```python
from build123d import *

# Parameters (mm, degrees)
SKETCH1_R           = 46.609
BOSS_EXTRUDE1_DEPTH = 38.1
SKETCH2_R           = 1.27
CUT_EXTRUDE1_DEPTH  = 38.1
SKETCH3_R           = 8.89
CUT_EXTRUDE2_DEPTH  = 38.1
SKETCH4_W           = 33.02
SKETCH4_H           = 33.02
CUT_EXTRUDE3_DEPTH  = 19.05
FILLET1_R           = 5.08


with BuildPart() as part:
    # Sketch1 → Boss-Extrude1 (new body)
    with BuildSketch(Plane(origin=(0, 0, 0), x_dir=(1, 0, 0), z_dir=(0, 1, 0))):
        Circle(SKETCH1_R)
    extrude(amount=BOSS_EXTRUDE1_DEPTH)

    # Sketch2 → Cut-Extrude1 (cut)
    with BuildSketch(Plane(origin=(0, 38.1, 0), x_dir=(1, 0, 0), z_dir=(0, 1, 0))):
        with Locations((12.7, 32.512)):
            Circle(SKETCH2_R)
        with Locations((-12.7, 32.512)):
            Circle(SKETCH2_R)
    extrude(amount=-CUT_EXTRUDE1_DEPTH, mode=Mode.SUBTRACT)

    # Sketch3 → Cut-Extrude2 (cut)
    with BuildSketch(Plane(origin=(0, 38.1, 0), x_dir=(1, 0, 0), z_dir=(0, 1, 0))):
        with Locations((-26.409958794, 0)):
            Circle(SKETCH3_R)
    extrude(amount=-CUT_EXTRUDE2_DEPTH, mode=Mode.SUBTRACT)

    # Sketch4 → Cut-Extrude3 (cut)
    with BuildSketch(Plane(origin=(0, 38.1, 0), x_dir=(1, 0, 0), z_dir=(0, 1, 0))):
        with Locations((16.51, 0)):
            Rectangle(SKETCH4_W, SKETCH4_H)
    extrude(amount=-CUT_EXTRUDE3_DEPTH, mode=Mode.SUBTRACT)

    # Fillet1
    fillet1_edges = [part.edges().sort_by_distance(p)[0] for p in [
        (0, 28.575, 16.51),
        (0, 28.575, -16.51),
        (33.02, 28.575, -16.51),
        (33.02, 28.575, 16.51),
    ]]
    fillet(fillet1_edges, radius=FILLET1_R)


solid = part.part
```
Source: CAD feature listing. Evaluate the final solid. Frame: model axes, mm. A direction names the side the tool comes from. Coordinates: 2 decimals unless noted, no trailing zeros. Loops run counter-clockwise (first coordinate to the right, second up) from the corner with the lowest first, then second, coordinate; pieces in that order, holes last. Notation, with made-up numbers: M -27,1 L 4,1 A23 ccw 4,12 Z; hole C -3,88 d11. An arc over 180 degrees is marked long. Use CSV: the item, a comma, the result in double quotes.
(1) Reachability of faces 1 (the face through (16, 19.05, 0)), 2 (the face through (13.911, 19.317, -32.893)) from +Z, -Z, +X, -X, +Y, -Y: full face, straight path, thin tool, end or side. Return the list, or none.
Answers follow:
face 1,"+Y"
face 2,"+Y, -Y"
(2) Line query: line 1 (X direction, y = 26, z = 0); line 2 (X direction, y = 23, z = -3); line 3 (Z direction, x = 12.7, y = 24.5). Output: solid intervals per line, ascending. Write a range as [from, to].
Answers follow:
line 1,"[-46.61, -35.3], [-17.52, 0], [33.02, 46.61]"
line 2,"[-46.51, -34.78], [-18.04, 0], [33.02, 46.51]"
line 3,"[-44.85, -33.78], [-31.24, -16.51], [16.51, 44.85]"
(3) Contact query for flat-ended pins moving along their axis: pin 1 (6 mm diameter, centred on y = 29.5, z = 13.5, fed in from -X); pin 2 (1.5 mm diameter, centred on x = 27.5, y = 8, fed in from +Z); pin 3 (2 mm diameter, centred on x = 34.5, y = 7, fed in from +Z). Output: stop coordinate, or through.
Answers follow:
pin 1,"x = -45.41"
pin 2,"z = 38.17"
pin 3,"z = 32.41"
(4) Cut plane D-D on x = -28. Return loops of the section in (y, z).
Answers follow:
outline,"M 0,-37.26 L 38.1,-37.26 L 38.1,-8.75 L 0,-8.75 Z; M 0,8.75 L 38.1,8.75 L 38.1,37.26 L 0,37.26 Z"
(5) Cut plane C-C on y = 23. Return loops of the section in (x, z).
Answers follow:
outline,"C 0,0 d93.22; hole C -26.41,0 d17.78; hole C -12.7,-32.51 d2.54; hole M 0,-11.43 A5.08 ccw 5.08,-16.51 L 27.94,-16.51 A5.08 ccw 33.02,-11.43 L 33.02,11.43 A5.08 ccw 27.94,16.51 L 5.08,16.51 A5.08 ccw 0,11.43 Z; hole C 12.7,-32.51 d2.54"
(6) Draft query along X for faces 3 (the face through (16, 29, -16.51)), 4 (the face through (-34.353, 18.783, -31.501)), 5 (the face through (-1, 0, -1)), 6 (the face through (31.571, 28.442, -14.982)). Return one class per face: pulls with the +X half, pulls with the -X half, needs draft (parallel to the pull), parting line crosses it, or undercut.
Answers follow:
face 3,"undercut"
face 4,"parting line crosses it"
face 5,"needs draft"
face 6,"undercut"
(7) Cut plane B-B on x = -12.7. Return loops of the section in (y, z).
Answers follow:
outline,"M 0,-44.85 L 38.1,-44.85 L 38.1,-33.78 L 0,-33.78 Z; M 0,-31.24 L 38.1,-31.24 L 38.1,44.85 L 0,44.85 Z"
(8) Cut plane A-A on z = 0. Return loops of the section in (x, y).
Answers follow:
outline,"M -46.61,0 L -35.3,0 L -35.3,38.1 L -46.61,38.1 Z; M -17.52,0 L 46.61,0 L 46.61,38.1 L 33.02,38.1 L 33.02,19.05 L 0,19.05 L 0,38.1 L -17.52,38.1 Z"
